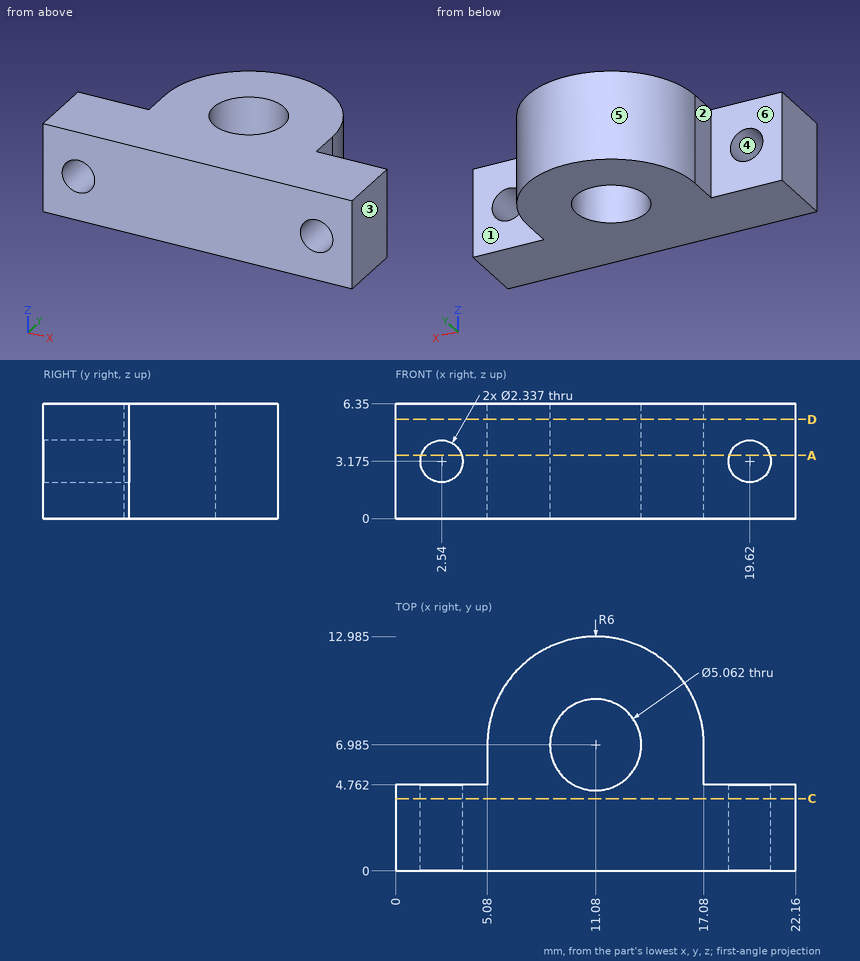
Verification items for this drawing (mm, ordinates from the low corner). A direction names the side the tool comes from. Give positions to 0.01 mm unless a question says otherwise; leave off trailing zeros. Loops run counter-clockwise (first coordinate to the right, second up) from the corner with the lowest first, then second, coordinate; pieces in that order, holes last. Notation, with made-up numbers: M 84,-26 L 98,-26 A16 ccw 98,-2 Z; hole C 55,37.5 d2. An arc over 180 degrees is marked long. Answer as a JSON object with one key per item and string values. Group by question number.
Item 1: Gauge pin test, flat end, axial feed: pin 1 (0.7 mm diameter, centred on y = 5.5, z = 1.5, fed in from -X). Record the tip position at first contact, or that the pin passes through.
Item 2: Sectioned sample at A-A on z = 3.5. Record the boundary of the cut face in (x, y) (1 decimal), plus the area to 3 significant figures.
Item 3: Sectioned sample at C-C on y = 4. Give the number of separate pieces and of enclosed holes in the cut face, plus the area to 3 significant figures.
Item 4: Access from +Z, -Z, +X, -X, +Y, -Y to the whole of each face (thin tool, end or side, straight path). Record for the marked faces 1, 2 and 3.
Item 5: Mould release check, pull along X, two halves, no side actions. Record for the marked faces 4, 5 and 6: pulls with the +X half, pulls with the -X half, needs draft (parallel to the pull), parting line crosses it, or undercut.
Item 6: Sectioned sample at D-D on z = 5.5. Record the boundary of the cut face in (x, y) (1 decimal), plus the area to 3 significant figures.
Item 7: Material ranges on L1, parallel to Y at x = 11.08, z = 4 (1 decimal); L2, parallel to Z at x = 19.62, y = 3.55; L3, parallel to X at y = 7.5, z = 1, recorded low to high.
Findings below:
{
 "1": {"pin 1": "x = 5.08"},
 "2": {"outline": "M 0,0 L 1.4,0 L 1.4,4.8 L 0,4.8 Z; M 3.7,0 L 18.5,0 L 18.5,4.8 L 17.1,4.8 L 17.1,7 A6 ccw 5.1,7 L 5.1,4.8 L 3.7,4.8 Z; M 20.7,0 L 22.2,0 L 22.2,4.8 L 20.7,4.8 Z; hole C 11.1,7 d5.1", "area": "147 mm2"},
 "3": {"separate pieces": "1", "enclosed holes": "2", "area": "132 mm2"},
 "4": {"face 1": "+Z, -Z, +X, +Y", "face 2": "+Z, -Z, -X, +Y", "face 3": "+Z, -Z, +X, +Y, -Y"},
 "5": {"face 4": "undercut", "face 5": "parting line crosses it", "face 6": "needs draft"},
 "6": {"outline": "M 0,0 L 22.2,0 L 22.2,4.8 L 17.1,4.8 L 17.1,7 A6 ccw 5.1,7 L 5.1,4.8 L 0,4.8 Z; hole C 11.1,7 d5.1", "area": "169 mm2"},
 "7": {"L1": "0 to 4.5, 9.5 to 13", "L2": "0 to 2.01, 4.34 to 6.35", "L3": "5.1 to 8.6, 13.56 to 17.06"}
}
